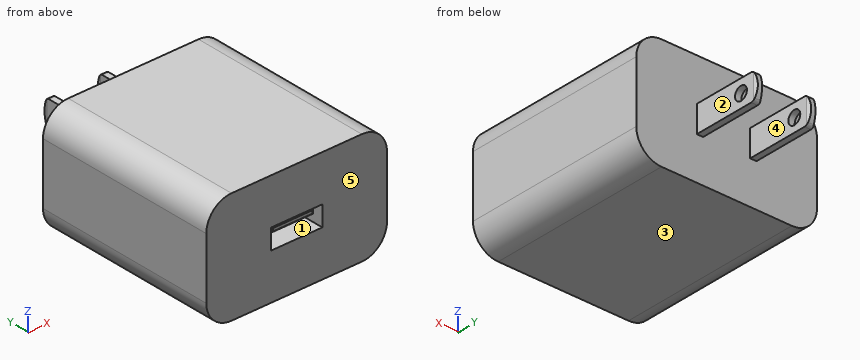
```python
from build123d import *

# Parameters (mm, degrees)
SKETCH2_W           = 43
SKETCH2_H           = 26.5
BOSS_EXTRUDE1_DEPTH = 44
SKETCH3_W           = 12.2
SKETCH3_H           = 4.8
CUT_EXTRUDE1_DEPTH  = 10
SKETCH4_W           = 1.5
SKETCH4_H           = 6.3
BOSS_EXTRUDE2_DEPTH = 16.2
SKETCH5_R           = 1.6
CUT_EXTRUDE2_DEPTH  = 16.2
CUT_EXTRUDE3_DEPTH  = 16.2
CUT_EXTRUDE4_DEPTH  = 16.2
FILLET1_R           = 1
FILLET2_R           = 6
SKETCH8_W           = 10.2
SKETCH8_H           = 1.5
BOSS_EXTRUDE3_DEPTH = 9
CHAMFER1_SIZE       = 0.4


with BuildPart() as part:
    # Sketch2 → Boss-Extrude1 (new body)
    with BuildSketch(Plane(origin=(0, 0, 0), x_dir=(1, 0, 0), z_dir=(0, 1, 0))):
        Rectangle(SKETCH2_W, SKETCH2_H)
    extrude(amount=BOSS_EXTRUDE1_DEPTH)

    # Sketch3 → Cut-Extrude1 (cut)
    with BuildSketch(Plane.XZ):
        Rectangle(SKETCH3_W, SKETCH3_H)
    extrude(amount=-CUT_EXTRUDE1_DEPTH, mode=Mode.SUBTRACT)

    # Sketch4 → Boss-Extrude2 (add)
    with BuildSketch(Plane(origin=(0, 44, 0), x_dir=(1, 0, 0), z_dir=(0, 1, 0))):
        with Locations((-6.35, 0)):
            Rectangle(SKETCH4_W, SKETCH4_H)
        with Locations((6.35, 0)):
            Rectangle(SKETCH4_W, SKETCH4_H)
    extrude(amount=BOSS_EXTRUDE2_DEPTH)

    # Sketch5 → Cut-Extrude2 (cut)
    with BuildSketch(Plane(origin=(7.1, 0, 0), x_dir=(0, 0, -1), z_dir=(1, 0, 0))):
        with Locations((0, 55.9)):
            Circle(SKETCH5_R)
    extrude(amount=-CUT_EXTRUDE2_DEPTH, mode=Mode.SUBTRACT)

    # Sketch6 → Cut-Extrude3 (cut)
    with BuildSketch(Plane(origin=(0, 0, -3.15), x_dir=(-1, 0, 0), z_dir=(0, 0, -1))):
        Polygon((-6.85, 60.2), (-5.85, 60.2), (-5.6, 59.231754163), (-5.6, 60.384988015), (-7.1, 60.384988015), (-7.1, 59.231754163), align=None)
    cut_extrude3 = extrude(amount=-CUT_EXTRUDE3_DEPTH, mode=Mode.SUBTRACT)

    # Mirror1: Cut-Extrude3 across plane
    add(cut_extrude3.mirror(Plane(origin=(0, 0, 0), x_dir=(0, 0, 1), z_dir=(1, 0, 0))), mode=Mode.SUBTRACT)

    # Sketch7 → Cut-Extrude4 (cut)
    with BuildSketch(Plane(origin=(7.1, 0, 0), x_dir=(0, 0, -1), z_dir=(1, 0, 0))):
        with BuildLine():
            Line((-3.15, 59.231754163), (-3.15, 61.207063701))
            Line((-3.15, 61.207063701), (3.15, 61.207063701))
            Line((3.15, 61.207063701), (3.15, 59.231754163))
            add(Edge.make_bspline(
                [(-3.15, 59.231754163), (0, 61.121756778), (3.15, 59.231754163)],
                knots=[0, 0, 0, 1, 1, 1], degree=2))
        make_face()
    extrude(amount=-CUT_EXTRUDE4_DEPTH, mode=Mode.SUBTRACT)

    # Fillet1
    fillet1_edges = [part.edges().sort_by_distance(p)[0] for p in [
        (6.35, 59.231754163, -3.15),
        (-6.35, 59.231754163, -3.15),
        (-6.35, 59.231754163, 3.15),
        (6.35, 59.231754163, 3.15),
    ]]
    fillet(fillet1_edges, radius=FILLET1_R)

    # Fillet2
    fillet2_edges = [part.edges().sort_by_distance(p)[0] for p in [
        (21.5, 22, 13.25),
        (-21.5, 22, 13.25),
        (-21.5, 22, -13.25),
        (21.5, 22, -13.25),
    ]]
    fillet(fillet2_edges, radius=FILLET2_R)

    # Sketch8 → Boss-Extrude3 (add)
    with BuildSketch(Plane.XZ.offset(-10)):
        with Locations((0, 0.95)):
            Rectangle(SKETCH8_W, SKETCH8_H)
    extrude(amount=BOSS_EXTRUDE3_DEPTH)

    # Chamfer1
    chamfer1_edges = [part.edges().sort_by_distance(p)[0] for p in [
        (0, 1, 1.7),
        (-5.1, 1, 0.95),
        (0, 1, 0.2),
        (5.1, 1, 0.95),
    ]]
    chamfer(chamfer1_edges, length=CHAMFER1_SIZE)


solid = part.part
```
Design review of the part built by this model. Coordinates are the model's own, in mm. Face numbers are marked on the shaded views. A direction names the side the tool comes from. Round coordinates to 2 decimals unless told otherwise and drop trailing zeros. Order: outer loops, then holes, each group sorted by start corner. A loop starts at its lowest first (then second) coordinate and runs counter-clockwise, first axis right, second up. Notation, with made-up numbers: (24.25, 10.25) - (42.25, 10.25) arc R22 ccw to (42.25, 45.25) - close; hole circle Ø9 at (25.25, 47). An arc over 180 degrees is marked (long way). Return JSON: item names as keys, results as strings.
Q1. Consider section B-B on x = 4. Write out the cut boundary in (y, z), plus the area to 3 significant figures.
Computed values:
{"outline": "(0, -13.25) - (44, -13.25) - (44, 13.25) - (0, 13.25) - (0, 2.4) - (10, 2.4) - (10, 1.7) - (1.4, 1.7) - (1, 1.3) - (1, 0.6) - (1.4, 0.2) - (10, 0.2) - (10, -2.4) - (0, -2.4) - close", "area": "1,130 mm2"}
Q2. Machinability: for the marked faces 4 and 5, which of the approach directions +Z, -Z, +X, -X, +Y, -Y give a long, thin tool a straight path to every point of the face, cutting with its end or side? Answer none if there is none.
Computed values:
{"face 4": "+Z, -Z, +Y", "face 5": "+Z, -Z, +X, -X, -Y"}
Q3. Consider section C-C on y = 55.9. Write out the cut boundary in (x, z), plus the area to 3 significant figures.
Computed values:
{"outline": "(-7.1, -3.15) - (-5.6, -3.15) - (-5.6, -1.6) - (-7.1, -1.6) - close; (-7.1, 1.6) - (-5.6, 1.6) - (-5.6, 3.15) - (-7.1, 3.15) - close; (5.6, -3.15) - (7.1, -3.15) - (7.1, -1.6) - (5.6, -1.6) - close; (5.6, 1.6) - (7.1, 1.6) - (7.1, 3.15) - (5.6, 3.15) - close", "area": "9.30 mm2"}
Q4. Consider section A-A on y = 45.5. Write out the cut boundary in (x, z).
Computed values:
{"outline": "(-7.1, -3.15) - (-5.6, -3.15) - (-5.6, 3.15) - (-7.1, 3.15) - close; (5.6, -3.15) - (7.1, -3.15) - (7.1, 3.15) - (5.6, 3.15) - close"}
Q5. For pin 1 Ø7 at (y, z) = (48.5, 1) entering from +X; pin 2 Ø0.5 at (x, y) = (6.5, 54.5) entering from -Z; pin 3 Ø8 at (x, z) = (-5.5, 1) entering from +Y; pin 4 Ø2.5 at (y, z) = (55.9, 0) entering from -X, all flat-tipped, find the tip position at first contact; note any pin that passes through.
Computed values:
{"pin 1": "stops at x = 7.1", "pin 2": "stops at z = -3.15", "pin 3": "stops at y = 60.18", "pin 4": "passes through"}
Q6. The part is to be moulded in two halves that separate along Z. For the marked faces 1, 2 and 3, say which applies: pulls with the +Z half, pulls with the -Z half, needs draft (parallel to the pull), parting line crosses it, or undercut.
Computed values:
{"face 1": "undercut", "face 2": "needs draft", "face 3": "pulls with the -Z half"}
Q7. Wall thickness on L1, parallel to Y at x = 6, z = 0; L2, parallel to Y at x = -6.6, z = 0; L3, parallel to Y at x = 19, z = 2.25: over which ranges is each line inside the solid? List them lowest first. Write a range as [from, to].
Computed values:
{"L1": "y = [10, 54.3], [57.5, 60.18]", "L2": "y = [0, 54.3], [57.5, 60.18]", "L3": "y = [0, 44]"}
Q8. Consider section D-D on z = 6.5. Write out the cut boundary in (x, y), plus the area to 3 significant figures.
Computed values:
{"outline": "(-21.5, 0) - (21.5, 0) - (21.5, 44) - (-21.5, 44) - close", "area": "1,890 mm2"}
